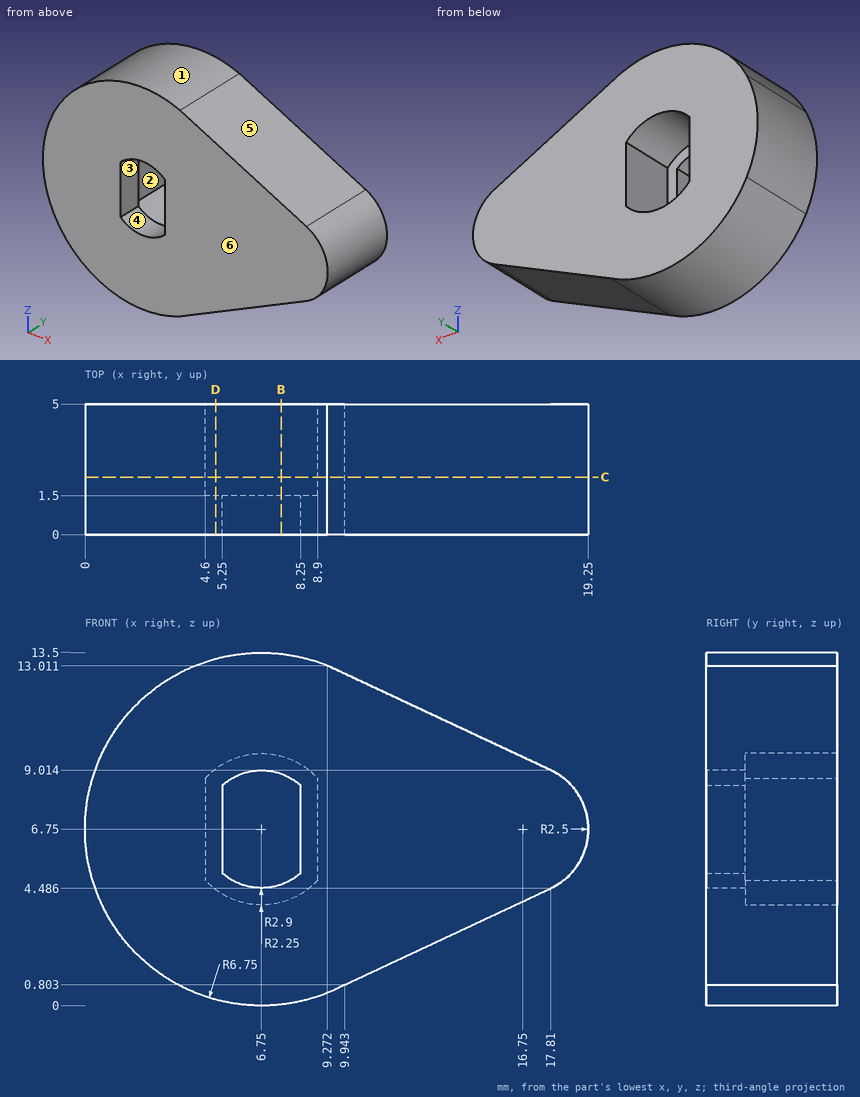
Answer from the drawing. Dimensions are ordinates in mm from the lowest x, y and z of the part. A direction names the side the tool comes from. Give positions to 0.01 mm unless a question says otherwise; leave off trailing zeros. Order: outer loops, then holes, each group sorted by start corner. A loop starts at its lowest first (then second) coordinate and runs counter-clockwise, first axis right, second up.
Item 1: The part is cut by section B-B, the plane x = 7.5. Give the vertices of the cut face in (y, z), and give its area (3 significant figures).
From the geometry:
outline: (0, 0.04) - (5, 0.04) - (5, 3.95) - (1.5, 3.95) - (1.5, 4.63) - (0, 4.63) - close; (0, 8.87) - (1.5, 8.87) - (1.5, 9.55) - (5, 9.55) - (5, 13.46) - (0, 13.46) - close
area: 41.1 mm2
Item 2: For a pull along X with two mould halves and no side action, classify the marked faces 3, 4, 5 and 6 as pulls with the +X half, pulls with the -X half, needs draft (parallel to the pull), parting line crosses it, or undercut.
From the geometry:
face 3: undercut
face 4: undercut
face 5: pulls with the +X half
face 6: needs draft
Item 3: Which of the six approach directions +Z, -Z, +X, -X, +Y, -Y give full straight-line access (tool end or side, diameter ignored) to the marked faces 1 and 2?
From the geometry:
face 1: +Z, +Y, -Y
face 2: +Y
Item 4: The part is cut by section D-D, the plane x = 5. Give the vertices of the cut face in (y, z), and give its area (3 significant figures).
From the geometry:
outline: (0, 0.23) - (5, 0.23) - (5, 4.44) - (1.5, 4.44) - (1.5, 9.06) - (5, 9.06) - (5, 13.27) - (0, 13.27) - close
area: 49.0 mm2
Item 5: Find the intervals of material crossed by probe 1 along Y at (x, z) = (8.5, 6.25); probe 2 along X at (y, z) = (2.95, 6.75); probe 3 along Z at (x, y) = (5, 4.2), in increasing order.
From the geometry:
probe 1: y = 0 to 1.5
probe 2: x = 0 to 4.6, 8.9 to 19.25
probe 3: z = 0.23 to 4.44, 9.06 to 13.27
Item 6: Given pin 1 Ø2 at (x, y) = (12, 3) entering from -Z; pin 2 Ø0.8 at (y, z) = (0.5, 7.5) entering from -X; pin 3 Ø1 at (x, y) = (15, 2) entering from +Z, each flat-ended and moving along its own axis, determine where each tip first touches the part or whether it passes through.
From the geometry:
pin 1: stops at z = 1.3
pin 2: stops at x = 0.01
pin 3: stops at z = 10.56
Item 7: The part is cut by section C-C, the plane y = 2.2. Give the vertices of the cut face in (x, z).
From the geometry:
outline: (9.27, 13.01) arc R6.75 ccw (long way) to (9.94, 0.8) - (17.81, 4.49) arc R2.5 ccw to (17.81, 9.01) - close; hole (4.6, 4.8) arc R2.9 ccw to (8.9, 4.8) - (8.9, 8.7) arc R2.9 ccw to (4.6, 8.7) - close
